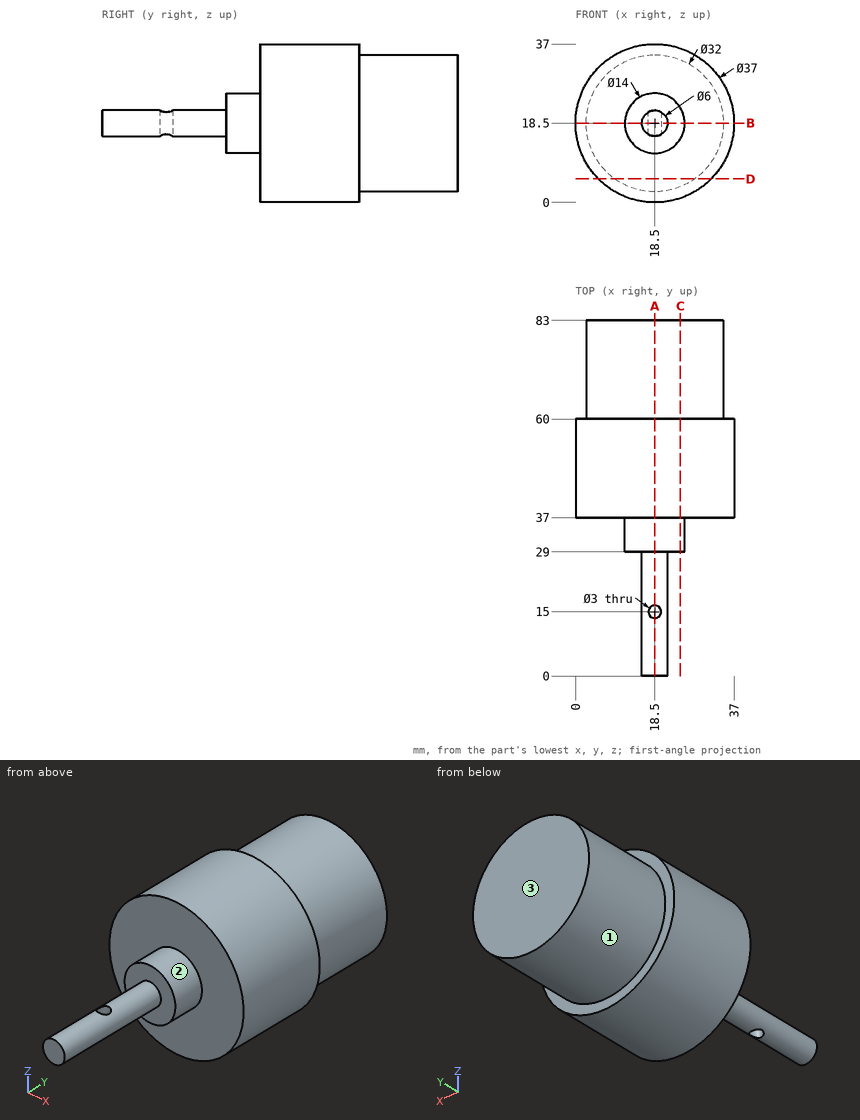
Design review of the part shown in the three views and the two pictorial views. Dimensions are in mm from the part's minimum x, y and z. A direction names the side the tool comes from. Round coordinates to 2 decimals unless told otherwise and drop trailing zeros. Loops run counter-clockwise (first coordinate to the right, second up) from the corner with the lowest first, then second, coordinate; pieces in that order, holes last. Notation, with made-up numbers: (5.25, -16.75) - (44.25, -16.75) arc R30 ccw to (44.25, 14.25) - close; hole circle Ø4 at (55.5, 88.5). An arc over 180 degrees is marked (long way). One line per item, written item: value. Start each with the question number.
Item 1: Clearance check with flat-ended pins moving along their axes: pin 1 Ø18.5 at (x, z) = (13, 20.5) entering from -Y; pin 2 Ø5 at (x, y) = (24, 52) entering from -Z; pin 3 Ø3 at (x, y) = (32.5, 35) entering from -Z; pin 4 Ø4 at (y, z) = (40, 16) entering from +X. State where each tip first meets the part, or that it passes through.
Item 2: For L1, parallel to Y at x = 18.5, z = 17.5; L2, parallel to Y at x = 18, z = 18; L3, parallel to Y at x = 28, z = 30.5, list the stretches that pass through material, from the lowest coordinate up.
Item 3: Take a section at A-A (x = 18.5). Give the boundary of the cut face in (y, z), plus the area to 4 significant figures.
Item 4: Take a section at B-B (z = 18.5). Give the boundary of the cut face in (x, y).
Item 5: Take a section at D-D (z = 5.5). Give the boundary of the cut face in (x, y), plus the area to 3 significant figures.
Item 6: Take a section at C-C (x = 24.5). Give the boundary of the cut face in (y, z), plus the area to 3 significant figures.
Item 7: For the marked faces 1, 2 and 3, list the 3-axis set-ups (+Z, -Z, +X, -X, +Y, -Y) from which the entire face can be reached by the end or side of a thin tool; tool diameter is ignored.
Answer below:
1. pin 1: stops at y = 0
1. pin 2: stops at z = 0.24
1. pin 3: passes through
1. pin 4: stops at x = 36.99
2. L1: y = 0 to 13.5, 16.5 to 83
2. L2: y = 0 to 13.59, 16.41 to 83
2. L3: y = 37 to 83
3. outline: (0, 15.5) - (13.5, 15.5) - (13.5, 21.5) - (0, 21.5) - close; (16.5, 15.5) - (29, 15.5) - (29, 11.5) - (37, 11.5) - (37, 0) - (60, 0) - (60, 2.5) - (83, 2.5) - (83, 34.5) - (60, 34.5) - (60, 37) - (37, 37) - (37, 25.5) - (29, 25.5) - (29, 21.5) - (16.5, 21.5) - close
3. area: 1,855 mm2
4. outline: (0, 37) - (11.5, 37) - (11.5, 29) - (15.5, 29) - (15.5, 0) - (21.5, 0) - (21.5, 29) - (25.5, 29) - (25.5, 37) - (37, 37) - (37, 60) - (34.5, 60) - (34.5, 83) - (2.5, 83) - (2.5, 60) - (0, 60) - close; hole circle Ø3 at (18.5, 15)
5. outline: (5.34, 37) - (31.66, 37) - (31.66, 60) - (27.83, 60) - (27.83, 83) - (9.17, 83) - (9.17, 60) - (5.34, 60) - close
5. area: 1,030 mm2
6. outline: (29, 14.89) - (37, 14.89) - (37, 1) - (60, 1) - (60, 3.67) - (83, 3.67) - (83, 33.33) - (60, 33.33) - (60, 36) - (37, 36) - (37, 22.11) - (29, 22.11) - close
6. area: 1,540 mm2
7. face 1: +Y
7. face 2: -Y
7. face 3: +Z, -Z, +X, -X, +Y
